from build123d import *

# Parameters (mm, degrees)
BOSS_EXTRUDE1_DEPTH = 10


with BuildPart() as part:
    # Sketch1 → Boss-Extrude1 (new body)
    with BuildSketch(Plane(origin=(0, 0, 0), x_dir=(1, 0, 0), z_dir=(0, 1, 0))):
        Polygon((-215, -118), (-215, -151), (215, -151), (215, -118), (205, -118), (205, -101), (205, -56), (215, -56), (215, 151), (-215, 151), (-215, -56), (-205, -56), (-205, -101), (-205, -118), align=None)
        with BuildLine():
            Line((-179.385227366, -72.32161442), (-203.75855493, -16.948417804))
            Line((-203.75855493, -16.948417804), (-147.92772859, 7.626342219))
            Line((-147.92772859, 7.626342219), (-91.123775094, -121.425239977))
            Line((-91.123775094, -121.425239977), (-146.954601434, -146))
            Line((-146.954601434, -146), (-171.327928998, -90.626803384))
            ThreePointArc((-171.327928998, -90.626803384), (-184.509172664, -85.502858086), (-179.385227366, -72.32161442))
        make_face(mode=Mode.SUBTRACT)
        with BuildLine():
            Line((-69.380969017, -146), (-126.184922514, -16.948417804))
            Line((-126.184922514, -16.948417804), (-70.354096174, 7.626342219))
            Line((-70.354096174, 7.626342219), (-45.98076861, -47.746854397))
            ThreePointArc((-45.98076861, -47.746854397), (-32.799524944, -52.870799695), (-37.923470242, -66.052043361))
            Line((-37.923470242, -66.052043361), (-13.550142678, -121.425239977))
            Line((-13.550142678, -121.425239977), (-69.380969017, -146))
        make_face(mode=Mode.SUBTRACT)
        with BuildLine():
            Line((19.11852712, -146), (-37.685426377, -16.948417804))
            Line((-37.685426377, -16.948417804), (18.145399963, 7.626342219))
            Line((18.145399963, 7.626342219), (42.518727527, -47.746854397))
            ThreePointArc((42.518727527, -47.746854397), (55.699971193, -52.870799695), (50.576025895, -66.052043361))
            Line((50.576025895, -66.052043361), (74.94935346, -121.425239977))
            Line((74.94935346, -121.425239977), (19.11852712, -146))
        make_face(mode=Mode.SUBTRACT)
        with BuildLine():
            Line((107.618023257, -146), (50.81406976, -16.948417804))
            Line((50.81406976, -16.948417804), (106.6448961, 7.626342219))
            Line((106.6448961, 7.626342219), (131.018223664, -47.746854397))
            ThreePointArc((131.018223664, -47.746854397), (144.19946733, -52.870799695), (139.075522033, -66.052043361))
            Line((139.075522033, -66.052043361), (163.448849597, -121.425239977))
            Line((163.448849597, -121.425239977), (107.618023257, -146))
        make_face(mode=Mode.SUBTRACT)
        with BuildLine():
            Line((-129.407841861, -9.626342219), (-186.211795357, 119.425239977))
            Line((-186.211795357, 119.425239977), (-130.380969017, 144))
            Line((-130.380969017, 144), (-106.007641453, 88.626803384))
            ThreePointArc((-106.007641453, 88.626803384), (-92.826397787, 83.502858086), (-97.950343085, 70.32161442))
            Line((-97.950343085, 70.32161442), (-73.577015521, 14.948417804))
            Line((-73.577015521, 14.948417804), (-129.407841861, -9.626342219))
        make_face(mode=Mode.SUBTRACT)
        with BuildLine():
            Line((-40.908345724, -9.626342219), (-97.71229922, 119.425239977))
            Line((-97.71229922, 119.425239977), (-41.88147288, 144))
            Line((-41.88147288, 144), (-17.508145316, 88.626803384))
            ThreePointArc((-17.508145316, 88.626803384), (-4.32690165, 83.502858086), (-9.450846948, 70.32161442))
            Line((-9.450846948, 70.32161442), (14.922480616, 14.948417804))
            Line((14.922480616, 14.948417804), (-40.908345724, -9.626342219))
        make_face(mode=Mode.SUBTRACT)
        with BuildLine():
            Line((47.591150413, -9.626342219), (-9.212803083, 119.425239977))
            Line((-9.212803083, 119.425239977), (46.618023257, 144))
            Line((46.618023257, 144), (70.991350821, 88.626803384))
            ThreePointArc((70.991350821, 88.626803384), (84.172594487, 83.502858086), (79.048649189, 70.32161442))
            Line((79.048649189, 70.32161442), (103.421976753, 14.948417804))
            Line((103.421976753, 14.948417804), (47.591150413, -9.626342219))
        make_face(mode=Mode.SUBTRACT)
        with BuildLine():
            Line((136.09064655, -9.626342219), (79.286693054, 119.425239977))
            Line((79.286693054, 119.425239977), (135.117519394, 144))
            Line((135.117519394, 144), (159.490846958, 88.626803384))
            ThreePointArc((159.490846958, 88.626803384), (172.672090624, 83.502858086), (167.548145326, 70.32161442))
            Line((167.548145326, 70.32161442), (191.92147289, 14.948417804))
            Line((191.92147289, 14.948417804), (136.09064655, -9.626342219))
        make_face(mode=Mode.SUBTRACT)
    extrude(amount=-BOSS_EXTRUDE1_DEPTH)


solid = part.part
Work out the finished part from the listing and answer in its coordinate system (mm). A direction names the side the tool comes from. Round coordinates to 2 decimals unless told otherwise and drop trailing zeros. Order: outer loops, then holes, each group sorted by start corner. A loop starts at its lowest first (then second) coordinate and runs counter-clockwise, first axis right, second up. Notation, with made-up numbers: M 34,8 L 60,8 A36 cw 60,47 Z; hole C 16.25,-13.5 d9. An arc over 180 degrees is marked long. One line per item, written item: value.
Q1. Find section C-C on x = 184.5. Write down the section's boundary in (y, z), then the cut area to 3 significant figures.
Derived:
outline: M -10,-151 L 0,-151 L 0,-31.81 L -10,-31.81 Z; M -10,-11.68 L 0,-11.68 L 0,151 L -10,151 Z
area: 2,820 mm²
Q2. Determine the mould class of faces 3 (the face through (-3, -10, -2)), 4 (the face through (151.09, -4.93, 93.35)) for opening direction Z: released by +Z, released by -Z, zero draft, split by the parting line, or undercut.
Derived:
face 3: zero draft
face 4: undercut
Q3. Straight lines are drawn through the part: line 1 (Z direction, x = -9, y = -3); line 2 (Z direction, x = -69.5, y = -1.5); line 3 (X direction, y = -7.75, z = 51). For each, find the intervals that lie inside material, in ascending order.
Derived:
line 1: -151 to -119.52, -118.94 to -88.41, -70.53 to -69.3, -4.42 to 4.32, 82.12 to 151
line 2: -151 to -131.84, -55.33 to -5.69, 145.73 to 151
line 3: -215 to -188.77, -122.12 to -111.2, -33.88 to -22.7, 54.62 to 65.8, 143.12 to 215
Q4. Find section D-D on z = 1.5. Give the number of separate pieces and of enclosed holes in the cut face, then the cut area to 3 significant figures.
Derived:
separate pieces: 9
enclosed holes: 0
area: 2,430 mm²
Q5. For faces 1 (the face through (18.31, -4.93, -131.54)), 2 (the face through (-210, -5, 56)), determine the directions among +Z, -Z, +X, -X, +Y, -Y from which every point of the face is accessible in a straight line to the end or side of a thin tool.
Derived:
face 1: +Y, -Y
face 2: -X, +Y, -Y
Q6. Find section B-B on x = 10.5. Write down the section's boundary in (y, z).
Derived:
outline: M -10,-151 L 0,-151 L 0,-128.1 L -10,-128.1 Z; M -10,-74.64 L 0,-74.64 L 0,-25 L -10,-25 Z; M -10,-13 L 0,-13 L 0,-4.26 L -10,-4.26 Z; M -10,126.42 L 0,126.42 L 0,151 L -10,151 Z
Q7. A flat-ended cylindrical pin translates along its axis: pin 1 (5 mm diameter, centred on y = -8.5, z = 108.5, fed in from +X). Find the tip coordinate at first contact, or state that the pin passes through.
Derived:
pin 1: x = 205
Q8. Find section A-A on z = -35. Write down the section's boundary in (x, y).
Derived:
outline: M -215,-10 L -149.05,-10 L -149.05,0 L -215,0 Z; M -82.4,-10 L -60.55,-10 L -60.55,0 L -82.4,0 Z; M 6.1,-10 L 27.95,-10 L 27.95,0 L 6.1,0 Z; M 94.6,-10 L 116.45,-10 L 116.45,0 L 94.6,0 Z; M 183.1,-10 L 215,-10 L 215,0 L 183.1,0 Z
